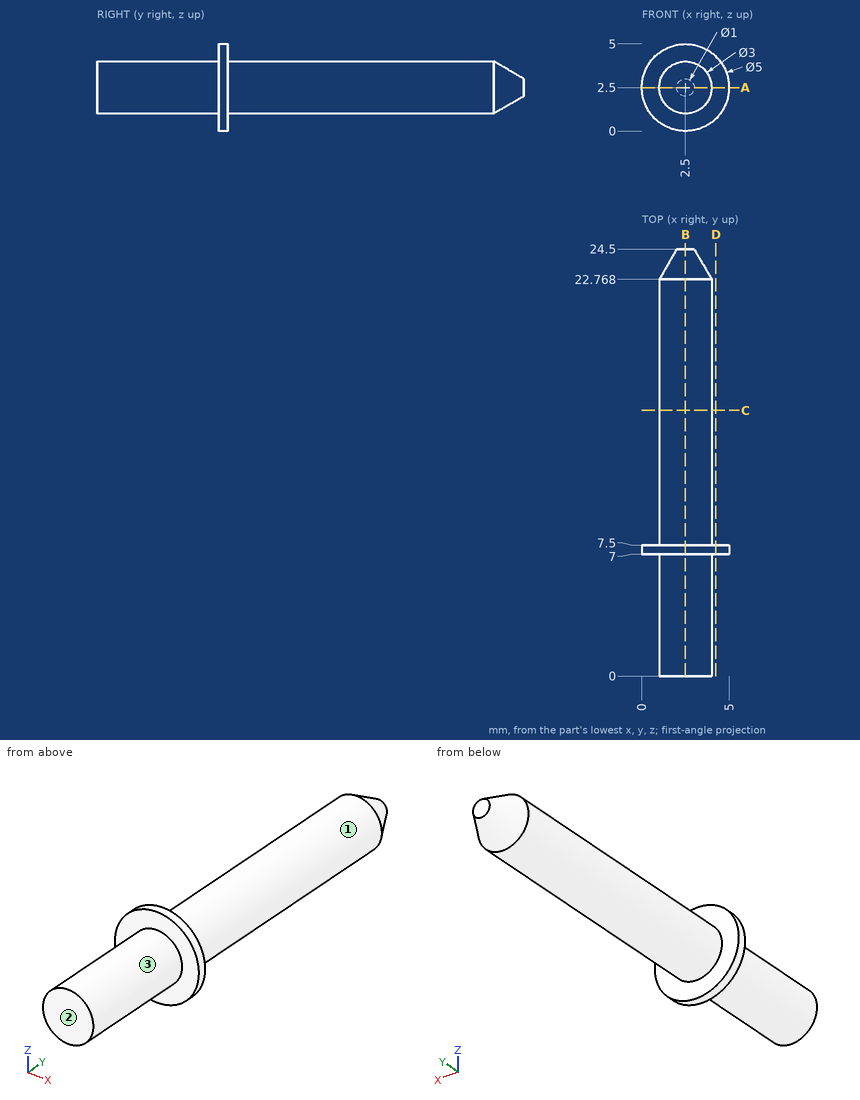
Answer from the drawing. Dimensions are ordinates in mm from the lowest x, y and z of the part. A direction names the side the tool comes from. Give positions to 0.01 mm unless a question says otherwise; leave off trailing zeros. Loops run counter-clockwise (first coordinate to the right, second up) from the corner with the lowest first, then second, coordinate; pieces in that order, holes last.
Item 1: A cutting plane is placed at B-B (x = 2.5). Give the vertices of the cut face in (y, z).
Derived:
outline: (0, 1) - (7, 1) - (7, 0) - (7.5, 0) - (7.5, 1) - (22.77, 1) - (24.5, 2) - (24.5, 3) - (22.77, 4) - (7.5, 4) - (7.5, 5) - (7, 5) - (7, 4) - (0, 4) - close
Item 2: A tool of negligible diameter and unlimited length cuts with its end or side. For the marked faces 1, 2 and 3, from which of +Z, -Z, +X, -X, +Y, -Y can it reach the whole face along a straight path? Write none if from no direction.
Derived:
face 1: +Y
face 2: +Z, -Z, +X, -X, -Y
face 3: -Y
Item 3: A cutting plane is placed at D-D (x = 4.25). Give the vertices of the cut face in (y, z).
Derived:
outline: (7, 0.71) - (7.5, 0.71) - (7.5, 4.29) - (7, 4.29) - close
Item 4: A cutting plane is placed at A-A (z = 2.5). Give the vertices of the cut face in (x, y).
Derived:
outline: (0, 7) - (1, 7) - (1, 0) - (4, 0) - (4, 7) - (5, 7) - (5, 7.5) - (4, 7.5) - (4, 22.77) - (3, 24.5) - (2, 24.5) - (1, 22.77) - (1, 7.5) - (0, 7.5) - close
Item 5: A cutting plane is placed at C-C (y = 15.25). Give the vertices of the cut face in (x, z), then the cut area to 3 significant figures.
Derived:
outline: circle Ø3 at (2.5, 2.5)
area: 7.07 mm2
Item 6: Each of these flat-tipped pins is pushed along its axis until it touches: pin 1 Ø1 at (x, y) = (1.5, 18.5) entering from +Z; pin 2 Ø3 at (y, z) = (13, 3.5) entering from +X; pin 3 Ø1.5 at (y, z) = (21.5, 1) entering from +X. Where does it stop, or does it pass through?
Derived:
pin 1: stops at z = 3.91
pin 2: stops at x = 4
pin 3: stops at x = 3.8
Item 7: Find the intervals of material crossed by line 1 along Y through (x, z) = (4.15, 1.7); line 2 along Z through (x, y) = (2.4, 8), in increasing order.
Derived:
line 1: y = 7 to 7.5
line 2: z = 1 to 4
